from build123d import *

# Parameters (mm, degrees)
F1_DEPTH    = 600
F2_R        = 4
F3_DEPTH    = 124
F5_W        = 150
F5_H        = 15
F6_DEPTH    = 3
F4_W        = 124
F4_H        = 55
F7_DEPTH    = 3
F8_T1_DEPTH = 271.3704583371


# Not quite as in the source:
# - a fillet or chamfer that OpenCascade refuses, or shapes differently, is made with other operations: its cross-section is extruded or revolved along the edge and cut away or added


with BuildPart() as f1:
    # F0 (on Front) → F1 (new body)
    with BuildSketch(Plane.XZ):
        Polygon((75, 17.5394031256), (75, 19.5394031256), (60, 19.5394031256), (60, -20.4605968744), (75, -20.4605968744), (75, -18.4605968744), (62, -18.4605968744), (62, 17.5394031256), align=None)
    extrude(amount=F1_DEPTH)


with BuildPart() as f1b:
    # F0 (on Front) → F1, piece 2 (new body)
    with BuildSketch(Plane.XZ):
        Polygon((-62, -18.4605968744), (-75, -18.4605968744), (-75, -20.4605968744), (-60, -20.4605968744), (-60, 19.5394031256), (-75, 19.5394031256), (-75, 17.5394031256), (-62, 17.5394031256), align=None)
    extrude(amount=F1_DEPTH)


with BuildPart() as f3_tool:
    # F2 (on face) → F3 (new body, through all)
    with BuildSketch(Plane.YZ.offset(62)):
        with Locations((-573.0000079556, -0.4398700211)):
            Circle(F2_R)
        with Locations((-534.0000079556, -0.4398700211)):
            Circle(F2_R)
        with Locations((-495.0000079556, -0.4398700211)):
            Circle(F2_R)
        with Locations((-456.0000079556, -0.4398700211)):
            Circle(F2_R)
        with Locations((-417.0000079556, -0.4398700211)):
            Circle(F2_R)
        with Locations((-378.0000079556, -0.4398700211)):
            Circle(F2_R)
        with Locations((-339.0000079556, -0.4398700211)):
            Circle(F2_R)
        with Locations((-300.0000079556, -0.4398700211)):
            Circle(F2_R)
        with Locations((-261.0000079556, -0.4398700211)):
            Circle(F2_R)
        with Locations((-222.0000079556, -0.4398700211)):
            Circle(F2_R)
        with Locations((-183.0000079556, -0.4398700211)):
            Circle(F2_R)
        with Locations((-144.0000079556, -0.4398700211)):
            Circle(F2_R)
        with Locations((-105.0000079556, -0.4398700211)):
            Circle(F2_R)
        with Locations((-66.0000079556, -0.4398700211)):
            Circle(F2_R)
        with Locations((-27.0000079556, -0.4398700211)):
            Circle(F2_R)
    extrude(amount=-F3_DEPTH)


with BuildPart() as f1_1:
    add(f1.part)

    # F3: cut by f3_tool
    add(f3_tool.part, mode=Mode.SUBTRACT)



with BuildPart() as f1b_1:
    add(f1b.part)

    # F3: cut by f3_tool
    add(f3_tool.part, mode=Mode.SUBTRACT)


with BuildPart() as f1_2:
    add(f1_1.part)

    add(f1b_1.part)  # F6 merges F1b
    # F5 (on face) → F6 (join)
    with BuildSketch(Plane(origin=(0, 0, -20.4605968744), x_dir=(1, 0, 0), z_dir=(0, 0, -1))):
        with Locations((0, 475.2312374115)):
            Rectangle(F5_W, F5_H)
        with Locations((0, 124.7687625885)):
            Rectangle(F5_W, F5_H)
    extrude(amount=F6_DEPTH)

    # F4 (on face) → F7 (join)
    with BuildSketch(Plane(origin=(0, 0, 0), x_dir=(-1, 0, 0), z_dir=(0, 1, 0))):
        with Locations((0, 7.0394031256)):
            Rectangle(F4_W, F4_H)
    extrude(amount=F7_DEPTH)

    # F8: chamfer of 5 x 28.3564090981 on 1 edges, made by hand

    # F8_s2 → F8_t1 (cut)
    with BuildSketch(Plane.YZ.offset(-135.6852291686)):
        Polygon((-25.3564090981, -20.4605968744), (3, -15.4605968744), (3, -20.4605968744), align=None)
    extrude(amount=F8_T1_DEPTH, mode=Mode.SUBTRACT)


solid = f1_2.part
Could you check a few things on this model? Use its own coordinates, in mm. A direction names the side the tool comes from. Give positions to 0.01 mm unless a question says otherwise; leave off trailing zeros. Write each loop counter-clockwise with the first axis right and the second up, starting at its lowest first coordinate (ties: lowest second). Pieces come first, ordered by that corner, then holes. Notation, with made-up numbers: (23, 54.25) -> (39, 54.25) arc R24 ccw to (39, 82.25) -> close; hole circle Ø1 at (50, -30). An arc over 180 degrees is marked (long way). Write each question's results on one line, items separated by ' | '. Start each with the question number.
Q1. Which directions (+Z, -Z, +X, -X, +Y, -Y) give clear straight access to the entire face, cutting with the end or side of a thin tool? Please do faces 1 (the face through (-68, -298, -20.461)), 2 (the face through (68, -72, -20.461)), 3 (the face through (68, -296, 17.539)), 4 (the face through (-69, -296, 17.539)), 5 (the face through (-68, -541, -20.461)).
Q2. I need wall thicknesses on probe 1 along X at (y, z) = (-497, -13); probe 2 along X at (y, z) = (-100, -20); probe 3 along Y at (x, z) = (-45, -12). Which ranges of each line are inside material? Lowest first, please.
Q3. Suppose I cut it at C-C, the plane z = 25.5. List the corners of the cut face in (x, y) for me, and give its area (3 significant figures).
Q4. Suppose I cut it at A-A, the plane x = 1. List the corners of the cut face in (y, z) for me.
Q5. Suppose I cut it at B-B, the plane y = -442. List the corners of the cut face in (x, z) for me, and give its area (3 significant figures).
Q6. I'm going to push flat-ended pins straight in: pin 1 Ø10.5 at (y, z) = (-456, -0.44) entering from -X; pin 2 Ø2 at (x, z) = (-30, 25.5) entering from -Y; pin 3 Ø14.5 at (x, y) = (-67.5, -421.5) entering from +Z; pin 4 Ø5 at (y, z) = (-105, -0.44) entering from -X. Where does each tip first touch, or does it pass through?
Q7. We'd pull the mould along X, two halves only. Please class faces 6 (the face through (69, -303, -18.461)), 7 (the face through (-1, -475, -20.461)): +X half, -X half, draft (parallel to the pull), parting line (faces both ways), or undercut.
Outcome:
1) face 1: -Z, +X, -X | face 2: -Z, +X, -X, +Y | face 3: +X, +Y, -Y | face 4: -X, +Y, -Y | face 5: -Z, +X, -X, -Y
2) probe 1: -62 to -60, 60 to 62 | probe 2: -75 to -60, 60 to 75 | probe 3: 0 to 3
3) outline: (-62, 0) -> (62, 0) -> (62, 3) -> (-62, 3) -> close | area: 372 mm2
4) outline: (-482.73, -23.46) -> (-467.73, -23.46) -> (-467.73, -20.46) -> (-482.73, -20.46) -> close; (-132.27, -23.46) -> (-117.27, -23.46) -> (-117.27, -20.46) -> (-132.27, -20.46) -> close; (0, -15.99) -> (3, -15.46) -> (3, 34.54) -> (0, 34.54) -> close
5) outline: (-75, -20.46) -> (-60, -20.46) -> (-60, 19.54) -> (-75, 19.54) -> (-75, 17.54) -> (-62, 17.54) -> (-62, -18.46) -> (-75, -18.46) -> close; (60, -20.46) -> (75, -20.46) -> (75, -18.46) -> (62, -18.46) -> (62, 17.54) -> (75, 17.54) -> (75, 19.54) -> (60, 19.54) -> close | area: 264 mm2
6) pin 1: x = -62 | pin 2: y = 0 | pin 3: z = 19.54 | pin 4: through
7) face 6: draft | face 7: undercut
